For this review, take the finished solid that the model builds, in its own axes (mm). A direction names the side the tool comes from. Coordinates: 2 decimals unless noted, no trailing zeros. Loops run counter-clockwise (first coordinate to the right, second up) from the corner with the lowest first, then second, coordinate; pieces in that order, holes last. Notation, with made-up numbers: (26, -18) - (75, -18) arc R20 cw to (75, 14) - close; hole circle Ø2 at (-34, -22.75). An arc over 180 degrees is marked (long way). Use one line per item in the form item = value. Start each with the question number.
1. Machinability: for faces 4 (the face through (197, 73, -1)), 5 (the face through (194.468, 2.465, -13.926)), 6 (the face through (181.857, 52.082, -24.155)), which of the approach directions +Z, -Z, +X, -X, +Y, -Y give a long, thin tool a straight path to every point of the face, cutting with its end or side? Answer none if there is none.
2. Add section A-A on x = 18. Give the boundary of the cut face in (y, z).
3. To check wall thickness, follow probe 1 along Y at (x, z) = (180.5, 0.5); probe 2 along Y at (x, z) = (8, 7); probe 3 along Z at (x, y) = (154, 71). State the ranges of each line that lie inside material, in increasing order.
4. For pin 1 Ø1.6 at (x, z) = (182, -12.5) entering from -Y; pin 2 Ø10.5 at (x, y) = (190.5, 103.5) entering from +Z; pin 3 Ø16.5 at (y, z) = (48.5, -6) entering from -X, all flat-tipped, find the tip position at first contact; note any pin that passes through.
5. Draft analysis for pull direction Z (two halves, no side actions). For faces 1 (the face through (188, 5, 0)), 2 (the face through (192, 110, -5)), 3 (the face through (185.67, 115.75, -23.25)), state which applies: +Z half, -Z half, draft (parallel to the pull), parting line (faces both ways), or undercut.
Autodesk Fusion 360 part; units mm, degrees
sketch "Sketch1" plane through (0, 0, 0) normal (0, 0, 1) x (1, 0, 0)
  line L0 (0, 0) -> (202, 0)
  line L1 (202, 0) -> (202, 116)
  line L2 (202, 116) -> (0, 116)
  line L3 (0, 116) -> (0, 0)
  dimension "d1" = 202
  dimension "d2" = 116
extrude "Extrude1" add sketch "Sketch1" along normal blind 5
sketch "Sketch2" plane through (0, 0, 0) normal (0, 0, -1) x (-1, 0, 0)
  circle A0 centre (-182, 107) radius 3.5
  line L0 (-182, 107) -> (-182, 9) construction
  line L1 (-182, 9) -> (-8, 9) construction
  circle A1 centre (-182, 9) radius 3.5
  line L2 (-8, 9) -> (-8, 107) construction
  circle A2 centre (-8, 9) radius 3.5
  circle A3 centre (-8, 107) radius 3.5
  line L3 (-8, 107) -> (-182, 107) construction
  line L4 (0, 0) -> (0, 116)
  line L5 (0, 116) -> (-202, 116)
  line L6 (-202, 116) -> (-202, 0)
  line L7 (-202, 0) -> (0, 0)
  dimension "d5" = 174
  dimension "d6" = 98
  dimension "d9" = 7
  dimension "d17" = 8
  dimension "d18" = 9
extrude "Extrude4" add sketch "Sketch2" against normal blind 11 contours A0 | A1 | A2 | A3
sketch "Sketch3" plane through (0, 0, 0) normal (0, -1, 0) x (1, 0, 0)
  line L0 (0, 0) -> (202, 0)
  line L1 (202, 0) -> (202, 5)
  line L2 (202, 5) -> (0, 5)
  line L3 (0, 5) -> (0, 0)
  circle A0 centre (185.5, -10.5) radius 16.5
  line L4 (202, -10.5) -> (202, 5)
  line L5 (169, -10.5) -> (169, 5)
  circle A1 centre (185.5, -10.5) radius 15.5
  dimension "d27" = 33
  dimension "d73" = 31
extrude "Extrude5" add sketch "Sketch3" against normal blind 116 contours L0 A0 L5 | L0 L2 A0 A1 | L0 A0 A1 | L0 A1 | L0 A1 | L0 A0 L4 | L0 L2 A0 A1
sketch "Sketch4" plane through (0, 0, 0) normal (0, -1, 0) x (1, 0, 0)
  line L0 (0, 0) -> (169, 0)
  line L1 (202, -10.5) -> (202, 5)
  line L2 (202, 5) -> (0, 5)
  line L3 (0, 5) -> (0, 0)
  circle A0 centre (185, -10) radius 10.25
  circle A1 centre (185, -10) radius 14.5
  line L4 (169, 0) -> (169, -10.5)
  arc A2 (169, -10.5) -> (202, -10.5) centre (185.5, -10.5) ccw
  dimension "d30" = 20.5
  dimension "d42" = 29
sketch "Sketch5" plane through (0, 0, 5) normal (0, 0, 1) x (-1, 0, 0)
  circle A0 centre (-8, -9) radius 3.5
  circle A1 centre (-8, -107) radius 3.5
  line L0 (0, -116) -> (0, 0)
  line L1 (0, 0) -> (-202, 0)
  line L2 (-202, -116) -> (0, -116)
  line L3 (-197, -13.5) -> (-182, -13.5)
  line L4 (-182, -13.5) -> (-182, -100.5)
  line L5 (-182, -100.5) -> (-197, -100.5)
  line L6 (-197, -100.5) -> (-197, -13.5)
  line L7 (-174.75, 0) -> (-195.25, 0)
  line L8 (-197, -100.5) -> (-187, -100.5)
  line L9 (-187, -100.5) -> (-187, -110)
  line L10 (-187, -110) -> (-197, -110)
  line L11 (-197, -110) -> (-197, -100.5)
  circle A2 centre (-182, -9) radius 3.5
  circle A3 centre (-182, -107) radius 3.5
  line L12 (-202, 0) -> (-202, -116)
  point P0 (-189.5, -100.5)
  dimension "d32" = 87
  dimension "d33" = 13.5
  dimension "d34" = 15
  dimension "d51" = 10
  dimension "d52" = 6
extrude "Extrude6" cut sketch "Sketch5" against normal blind 20.5 contours L3 L4 L5 L6 L8 | L5 L8 L9 L10 L11
extrude "Extrude7" cut sketch "Sketch4" against normal blind 95.5 from surface at -5 contours A0 | A1
sketch "Sketch6" plane through (0, 13.5, 0) normal (0, 1, 0) x (-1, 0, 0)
  line L0 (-197, 5) -> (-197, -1.8606)
  line L1 (-169, 0) -> (0, 0)
  line L2 (0, 0) -> (0, 5)
  line L3 (0, 5) -> (-202, 5)
  line L4 (-202, 5) -> (-202, -10.5)
  arc A0 (-202, -10.5) -> (-169, -10.5) centre (-185.5, -10.5) ccw
  circle A1 centre (-185.5, -10.5) radius 15
  line L5 (-169, -10.5) -> (-169, 0)
  line L6 (-182, 4.1863) -> (-182, 5)
  arc A2 (-182, 4.1863) -> (-197, -1.8606) centre (-185, -10) ccw
  line L7 (-182, 5) -> (-197, 5)
  dimension "d39" = 30
extrude "Extrude9" cut sketch "Sketch4" against normal blind 33 contours A0
fillet "Fillet2" radius 12.5 1 edges at (169, 58, 0)
sketch "Sketch7" plane through (0, 0, 5) normal (0, 0, 1) x (-1, 0, 0)
  circle A0 centre (-8, -9) radius 3.5
  circle A1 centre (-8, -107) radius 3.5
  line L0 (0, -116) -> (0, 0)
  line L1 (0, 0) -> (-202, 0)
  line L2 (-202, -116) -> (0, -116)
  line L3 (-187, -100.5) -> (-187, -110)
  line L4 (-187, -110) -> (-197, -110)
  line L5 (-197, -110) -> (-197, -100.5)
  line L6 (-197, -13.5) -> (-182, -13.5)
  line L7 (-182, -100.5) -> (-187, -100.5)
  circle A2 centre (-182, -107) radius 3.5
  line L8 (-202, 0) -> (-202, -116)
  line L9 (-182, -13.5) -> (-182, -100.5)
  circle A3 centre (-182, -9) radius 3.5
  line L10 (-197, -100.5) -> (-197, -13.5)
sketch "Sketch8" plane through (0, 0, 5) normal (0, 0, 1) x (-1, 0, 0)
  circle A0 centre (-90, -49.5) radius 8.5
  line L0 (0, -116) -> (0, 0)
  line L1 (0, 0) -> (-202, 0)
  dimension "d53" = 17
  dimension "d54" = 90
  dimension "d55" = 49.5
extrude "Extrude10" add sketch "Sketch8" along normal blind 6.4
fillet "Fillet3" radius 2 1 edges at (97.9248, 46.4263, 5)
sketch "Sketch9" plane through (0, 0, 0) normal (0, 0, -1) x (1, 0, 0)
  line L0 (156.569, 0) -> (0, 0)
  line L1 (0, 0) -> (0, -116)
  line L2 (0, -116) -> (156.569, -116)
  line L3 (6.3834, -104.2) -> (4.7668, -107)
  line L4 (4.7668, -107) -> (6.3834, -109.8)
  line L5 (6.3834, -109.8) -> (9.6166, -109.8)
  line L6 (9.6166, -109.8) -> (11.2332, -107)
  line L7 (11.2332, -107) -> (9.6166, -104.2)
  line L8 (9.6166, -104.2) -> (6.3834, -104.2)
  line L9 (6.3834, -6.2) -> (4.7668, -9)
  line L10 (4.7668, -9) -> (6.3834, -11.8)
  line L11 (6.3834, -11.8) -> (9.6166, -11.8)
  line L12 (9.6166, -11.8) -> (11.2332, -9)
  line L13 (11.2332, -9) -> (9.6166, -6.2)
  line L14 (9.6166, -6.2) -> (6.3834, -6.2)
  line L15 (178.7668, -107) -> (180.3834, -109.8)
  line L16 (180.3834, -109.8) -> (183.6166, -109.8)
  line L17 (183.6166, -109.8) -> (185.2332, -107)
  line L18 (185.2332, -107) -> (183.6166, -104.2)
  line L19 (183.6166, -104.2) -> (180.3834, -104.2)
  line L20 (180.3834, -104.2) -> (178.7668, -107)
  line L21 (183.6166, -6.2) -> (180.3834, -6.2)
  line L22 (180.3834, -6.2) -> (178.7668, -9)
  line L23 (178.7668, -9) -> (180.3834, -11.8)
  line L24 (180.3834, -11.8) -> (183.6166, -11.8)
  line L25 (183.6166, -11.8) -> (185.2332, -9)
  line L26 (185.2332, -9) -> (183.6166, -6.2)
  line L27 (156.569, -116) -> (156.569, 0)
  line L28 (156.569, -116) -> (156.569, 0)
  line L29 (156.569, 0) -> (0, 0)
  line L30 (0, 0) -> (0, -116)
  line L31 (0, -116) -> (156.569, -116)
  point P0 (8, -107)
  point P1 (8, -9)
  point P2 (182, -107)
  point P3 (182, -107)
  point P4 (182, -9)
  point P5 (182, -9)
  dimension "d60" = 5.6
chamfer "Chamfer3" distance 3 angle 45 2 edges at (0, 116, 2.5) (0, 0, 2.5)
chamfer "Chamfer4" distance 4 angle 45 11 edges at (0, 58, 0) (79.7845, 0, 0) (165.0977, 0, -3.3615) (186.0693, 0, -26.9902) (202, 0, -2.75) (1.5, 1.5, 0) (1.5, 114.5, 0) (79.7845, 116, 0) (165.0977, 116, -3.3615) (186.0693, 116, -26.9902) (202, 116, -2.75)
hole "Hole1" at (182, 9, 0) at (182, 107, 0) at (8, 107, 0) at (8, 9, 0) direction (0, 0, 1) diameter 3.4 end through all
extrude "Extrude11" cut sketch "Sketch9" along normal blind 50 and the other way blind 3.5 contours L3 L4 L5 L6 L7 L8 | L9 L10 L11 L12 L13 L14 | L15 L16 L17 L18 L19 L20 | L21 L22 L23 L24 L25 L26
Conclusion:
q1.face_4 = +Z
q1.face_5 = -Y
q1.face_6 = none
q2.outline = (0, 4) - (4, 0) - (112, 0) - (116, 4) - (116, 5) - (0, 5) - close
q3.probe_1 = 0 to 5, 100.5 to 104.2, 109.8 to 116
q3.probe_2 = 5.5 to 7.3, 10.7 to 12.5, 103.5 to 105.3, 108.7 to 110.5
q3.probe_3 = 0 to 5
q4.pin_1 = 100.5
q4.pin_2 = 5
q4.pin_3 = 1.75
q5.face_1 = undercut
q5.face_2 = draft
q5.face_3 = -Z half
